Part model, mm, in its own coordinate system. Face numbers are marked on the shaded views. A direction names the side the tool comes from. Round coordinates to 2 decimals unless told otherwise and drop trailing zeros. Order: outer loops, then holes, each group sorted by start corner. A loop starts at its lowest first (then second) coordinate and runs counter-clockwise, first axis right, second up. Notation, with made-up numbers: (35, -8) - (47, -8) arc R29 cw to (47, 26) - close; hole circle Ø10 at (79.5, -23). An arc over 180 degrees is marked (long way). Answer as a JSON object with one key per item and string values.
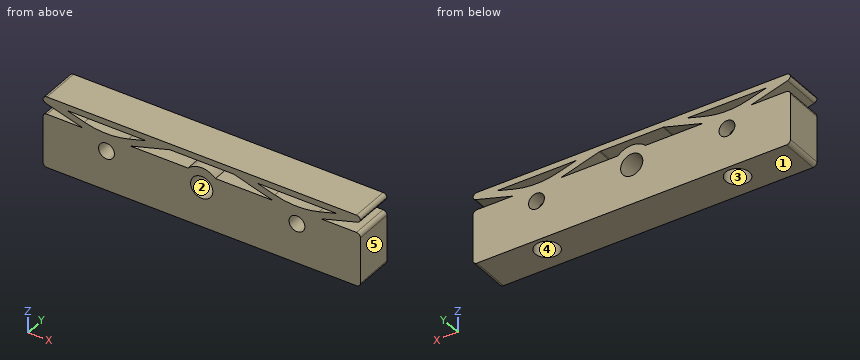
```python
from build123d import *

# Parameters (mm, degrees)
SKETCH1_W               = 40
SKETCH1_H               = 9
BOSS_EXTRUDE1_DEPTH     = 5
CUT_EXTRUDE1_DEPTH      = 5
CUT_EXTRUDE1_DEPTH_BACK = 10
SKETCH2_R               = 1
SKETCH2_R_2             = 1.4
FILLET1_R               = 10
FILLET2_R               = 0.5
SKETCH3_R               = 1.5
CUT_EXTRUDE6_DEPTH      = 3.8
SKETCH4_W               = 3
SKETCH4_H               = 0.5
CUT_EXTRUDE7_DEPTH      = 2.5


with BuildPart() as part:
    # Sketch1 → Boss-Extrude1 (new body)
    with BuildSketch(Plane(origin=(0, 0, 0), x_dir=(1, 0, 0), z_dir=(0, 1, 0))):
        with Locations((20, 4.5)):
            Rectangle(SKETCH1_W, SKETCH1_H)
    extrude(amount=BOSS_EXTRUDE1_DEPTH)

    # Sketch2 → Cut-Extrude1 (cut, two sides: drawn at the far end of the back side and taken through both)
    with BuildSketch(Plane(origin=(0, 5, 0), x_dir=(1, 0, 0), z_dir=(0, 1, 0)).offset(-CUT_EXTRUDE1_DEPTH_BACK)):
        with Locations(Location((8, 4, 0), (0, 0, 90))):
            Circle(SKETCH2_R)
        with Locations(Location((32, 4, 0), (0, 0, 90))):
            Circle(SKETCH2_R)
        with Locations(Location((20, 4, 0), (0, 0, 90))):
            Circle(SKETCH2_R_2)
        with BuildLine():
            ThreePointArc((21.734935157, 2.2), (20, 1.5), (18.265064843, 2.2))
            Line((18.265064843, 2.2), (11, 2.2))
            Line((11, 2.2), (16, 0.75))
            Line((16, 0.75), (24, 0.75))
            Line((24, 0.75), (29, 2.2))
            Line((29, 2.2), (21.734935157, 2.2))
        make_face()
        Polygon((13, 0.75), (8, 2.2), (3, 0.75), align=None)
        Polygon((37, 0.75), (32, 2.2), (27, 0.75), align=None)
        Polygon((0, 0.75), (5, 2.2), (0, 2.2), align=None)
        Polygon((40, 2.2), (35, 2.2), (40, 0.75), align=None)
    extrude(amount=CUT_EXTRUDE1_DEPTH + CUT_EXTRUDE1_DEPTH_BACK, mode=Mode.SUBTRACT)

    # Fillet1
    fillet1_edges = [part.edges().sort_by_distance(p)[0] for p in [
        (32, 2.5, -2.2),
        (8, 2.5, -2.2),
    ]]
    fillet(fillet1_edges, radius=FILLET1_R)

    # Fillet2
    # the kernel refuses this fillet: 0.5 mm, written as the material it adds along each edge
    with BuildSketch(Plane(origin=(24, 5, -0.75), x_dir=(0.9604291387787307, 0, -0.27852445024583705), z_dir=(0, -1, 0))) as fillet2_piece_1:
        with BuildLine():
            CenterArc((FILLET2_R * 0.142073204655, -FILLET2_R), FILLET2_R, 90, 16.172159016)
            Line((-FILLET2_R * 0.136451245591, -FILLET2_R * 0.0395708612213), (0, 0))
            Line((0, 0), (FILLET2_R * 0.142073204655, 0))
        make_face()
    extrude(amount=5)
    with BuildSketch(Plane(origin=(16, 0, -0.75), x_dir=(1, 0, 0), z_dir=(0, 1, 0))) as fillet2_piece_2:
        with BuildLine():
            CenterArc((FILLET2_R * 0.142073204655, FILLET2_R), FILLET2_R, 253.827840984, 16.172159016)
            Line((-FILLET2_R * 0.136451245591, FILLET2_R * 0.0395708612213), (0, 0))
            Line((0, 0), (FILLET2_R * 0.142073204655, 0))
        make_face()
    extrude(amount=5)
    # the kernel refuses this fillet: 0.5 mm, written as the material it takes off along each edge
    with BuildSketch(Plane(origin=(0, 5.939001537, -0.75), x_dir=(0.960429138778732, 0, -0.2785244502458324), z_dir=(0, -1, 0)), Plane(origin=(40, 5.939001537, -0.75), x_dir=(0, 0, 1), z_dir=(0, -1, 0))) as fillet2_2_piece_1:
        with BuildLine():
            CenterArc((FILLET2_R * 0.75120122935, FILLET2_R), FILLET2_R, 196.172159016, 73.827840984)
            Line((-FILLET2_R * 0.209227909429, FILLET2_R * 0.721475549754), (0, 0))
            Line((0, 0), (FILLET2_R * 0.75120122935, 0))
        make_face()
    extrude(amount=6.878003073, mode=Mode.SUBTRACT)
    with BuildSketch(Plane(origin=(0, 6.25, -2.2), x_dir=(0, 0, -1), z_dir=(0, -1, 0)), Plane(origin=(40, 6.25, -2.2), x_dir=(-1, 0, 0), z_dir=(0, -1, 0)), Plane(origin=(0, -1.25, 0), x_dir=(1, 0, 0), z_dir=(0, 1, 0))) as fillet2_2_piece_2:
        with BuildLine():
            CenterArc((FILLET2_R, FILLET2_R), FILLET2_R, 180, 90)
            Line((0, FILLET2_R), (0, 0))
            Line((0, 0), (FILLET2_R, 0))
        make_face()
    extrude(amount=7.5, mode=Mode.SUBTRACT)
    with BuildSketch(Plane(origin=(0, -1.25, -9), x_dir=(1, 0, 0), z_dir=(0, 1, 0)), Plane(origin=(40, -1.25, -9), x_dir=(0, 0, 1), z_dir=(0, 1, 0)), Plane(origin=(40, -1.25, 0), x_dir=(-1, 0, 0), z_dir=(0, 1, 0))) as fillet2_2_piece_3:
        with BuildLine():
            CenterArc((FILLET2_R, -FILLET2_R), FILLET2_R, 90, 90)
            Line((0, -FILLET2_R), (0, 0))
            Line((0, 0), (FILLET2_R, 0))
        make_face()
    extrude(amount=7.5, mode=Mode.SUBTRACT)

    # Sketch3 → Cut-Extrude6 (cut)
    with BuildSketch(Plane(origin=(0, 0, -9), x_dir=(-1, 0, 0), z_dir=(0, 0, -1))):
        with Locations((-32, 3)):
            Circle(SKETCH3_R)
        with Locations((-8, 3)):
            Circle(SKETCH3_R)
    extrude(amount=-CUT_EXTRUDE6_DEPTH, mode=Mode.SUBTRACT)

    # Sketch4 → Cut-Extrude7 (cut)
    with BuildSketch(Plane(origin=(0, 0, -5.2), x_dir=(-1, 0, 0), z_dir=(0, 0, -1))):
        with Locations((-32, 3)):
            Rectangle(SKETCH4_W, SKETCH4_H)
        with Locations((-8, 3)):
            Rectangle(SKETCH4_W, SKETCH4_H)
    extrude(amount=-CUT_EXTRUDE7_DEPTH, mode=Mode.SUBTRACT)


solid = part.part
```
Item 1: Tool access for the marked faces 4 and 5: list every direction of +Z, -Z, +X, -X, +Y, -Y with a clear straight run to the whole face (end or side of a thin tool).
Taken from the geometry:
{"face 4": "-Z", "face 5": "+Z, -Z, +X, +Y, -Y"}
Item 2: Cut at A-A (x = 25). Write the cut outline in (y, z), plus the area to 3 significant figures.
Taken from the geometry:
{"outline": "(0, -9) - (5, -9) - (5, -2.2) - (0, -2.2) - close; (0, -1.04) - (5, -1.04) - (5, 0) - (0, 0) - close", "area": "39.2 mm2"}
Item 3: Cut at B-B (z = -4). State how many separate pieces and enclosed holes the cut face has, plus the area to 3 significant figures.
Taken from the geometry:
{"separate pieces": "4", "enclosed holes": "0", "area": "165 mm2"}
Item 4: Cut at D-D (x = 32). Write the cut outline in (y, z), plus the area to 3 significant figures.
Taken from the geometry:
{"outline": "(0, -9) - (1.5, -9) - (1.5, -5.2) - (2.75, -5.2) - (2.75, -5) - (0, -5) - close; (0, -3) - (2.75, -3) - (2.75, -2.7) - (3.25, -2.7) - (3.25, -3) - (5, -3) - (5, -1.79) - (0, -1.79) - close; (0, -0.75) - (5, -0.75) - (5, 0) - (0, 0) - close; (3.25, -5.2) - (4.5, -5.2) - (4.5, -9) - (5, -9) - (5, -5) - (3.25, -5) - close", "area": "18.2 mm2"}
Item 5: Probe L1, parallel to Z at x = 32, y = 2.05; L2, parallel to X at y = 0.8, z = -4; L3, parallel to X at y = 3.05, z = -8. List the from-to ranges inside material, lowest first. Write a range as from..to.
Taken from the geometry:
{"L1": "-5.2..-5, -3..-1.79, -0.75..0", "L2": "0..7, 9..18.6, 21.4..31, 33..40", "L3": "0..6.5, 9.5..30.5, 33.5..40"}
Item 6: Cut at C-C (x = 20). Write the cut outline in (y, z).
Taken from the geometry:
{"outline": "(0, -9) - (5, -9) - (5, -5.4) - (0, -5.4) - close; (0, -2.6) - (5, -2.6) - (5, -1.5) - (0, -1.5) - close; (0, -0.75) - (5, -0.75) - (5, 0) - (0, 0) - close"}
Item 7: Two-plate mould, pull along Z, no slides. Class the marked faces 1, 2 and 3: pulls with the +Z half, pulls with the -Z half, needs draft (parallel to the pull), parting line crosses it, or undercut.
Taken from the geometry:
{"face 1": "pulls with the -Z half", "face 2": "undercut", "face 3": "needs draft"}
Item 8: Drop flat-ended pins along their axis: P1, Ø1.6, axis at x = 32, z = -4, coming from the +Y side (3 decimals); P2, Ø1.4, axis at x = 32, y = 3.5, coming from the -Z side. Give the stop position or say it passes through.
Taken from the geometry:
{"P1": "through", "P2": "z = -5.2"}
